Read the model definition and answer for the solid it produces. Units are mm, in the model's axes. Face numbers are marked on the shaded views. A direction names the side the tool comes from. Coordinates: 2 decimals unless noted, no trailing zeros. Write each loop counter-clockwise with the first axis right and the second up, starting at its lowest first coordinate (ties: lowest second). Pieces come first, ordered by that corner, then holes. Notation, with made-up numbers: (37, -21.5) -> (58, -21.5) arc R20 cw to (58, 6.5) -> close; hole circle Ø6 at (-30.75, 72). An arc over 180 degrees is marked (long way). One line per item, written item: value. Start each with the question number.
1. Find section C-C, the plane y = 7.5. State how many separate pieces and enclosed holes the cut face has, and give its area (3 significant figures).
2. Find section D-D, the plane x = -21.5. Write down the section's boundary in (y, z).
3. Find section B-B, the plane x = 0. Write down the section's boundary in (y, z), and give its area (3 significant figures).
4. Find section A-A, the plane z = -115. Write down the section's boundary in (x, y), and give its area (3 significant figures).
5. For a pull along Z with two mould halves and no side action, classify the marked faces 1, 2 and 3 as pulls with the +Z half, pulls with the -Z half, needs draft (parallel to the pull), parting line crosses it, or undercut.
6. Given P1, Ø1, axis at y = 7, z = -140.5, coming from the -X side; P2, Ø1, axis at x = 2.5, y = 4.5, coming from the -Z side; P3, Ø18, axis at x = 0, z = -150, coming from the -Y side; P4, Ø5, axis at y = 6.5, z = -125, coming from the +X side, each flat-ended and moving along its own axis, determine where each tip first touches the part or whether it passes through.
7. For the marked faces 4 and 5, determine the directions among +Z, -Z, +X, -X, +Y, -Y from which every point of the face is accessible in a straight line to the end or side of a thin tool.
8. Consider line 1 along X through (y, z) = (3.75, -150); line 2 along Z through (x, y) = (-12.5, 5.25); line 3 along X through (y, z) = (2, -59.5). Determine where each line is inside the solid, lowest interval first.
```python
from build123d import *

# Parameters (mm, degrees)
SKETCH_1_R               = 5
SKETCH_1_R_2             = 15
EXTRUDE_1_DEPTH          = 12
FILLET_1_R               = 3
SKETCH_2_R               = 2
CUT_EXTRUDE_1_DEPTH      = 179.881245523
PATTERN_CIRCULAR_3_COUNT = 2
PATTERN_CIRCULAR_3_ANGLE = 50
PATTERN_CIRCULAR_4_COUNT = 2
PATTERN_CIRCULAR_4_ANGLE = 50


with BuildPart() as part:
    # 草图1 → 凸台-拉伸1 (new body)
    with BuildSketch(Plane(origin=(0, 0, 0), x_dir=(1, 0, 0), z_dir=(0, 1, 0))):
        with BuildLine():
            Line((-17.971076762, -1.02), (-26.457418567, 148.498333333))
            ThreePointArc((-26.457418567, 148.498333333), (0, 176.5), (26.457418567, 148.498333333))
            Line((26.457418567, 148.498333333), (17.971076762, -1.02))
            ThreePointArc((17.971076762, -1.02), (0, -18), (-17.971076762, -1.02))
        make_face()
        with Locations(Location((0, 0, 0), (0, 0, 270))):
            Circle(SKETCH_1_R, mode=Mode.SUBTRACT)
        with Locations(Location((0, 150, 0), (0, 0, 270))):
            Circle(SKETCH_1_R_2, mode=Mode.SUBTRACT)
        Polygon((-12.740980954, 12.714849757), (-18.554385191, 115.139490738), (10.712851955, 17.329399023), align=None, mode=Mode.SUBTRACT)
        Polygon((13.283215706, 22.268322657), (18.830257334, 120), (-12, 127), align=None, mode=Mode.SUBTRACT)
    extrude(amount=EXTRUDE_1_DEPTH)

    # 圆角1
    fillet_1_edges = [part.edges().sort_by_distance(p)[0] for p in [
        (-12.740980954, 6, -12.714849757),
        (10.712851955, 6, -17.329399023),
        (-18.554385191, 6, -115.139490738),
        (18.830257334, 6, -120),
        (-12, 6, -127),
        (13.283215706, 6, -22.268322657),
    ]]
    fillet(fillet_1_edges, radius=FILLET_1_R)

    # 草图2 → 切除-拉伸1 (cut, through all)
    with BuildSketch(Plane(origin=(0, 12, 0), x_dir=(1, 0, 0), z_dir=(0, 1, 0))):
        with Locations(Location((-21.5, 150, 0), (0, 0, 270))):
            Circle(SKETCH_2_R)
        with Locations(Location((21.5, 150, 0), (0, 0, 270))):
            Circle(SKETCH_2_R)
    cut_extrude_1 = extrude(amount=-CUT_EXTRUDE_1_DEPTH, mode=Mode.SUBTRACT)

    # 阵列(圆周)3: 切除-拉伸1 ×2 about axis
    pattern_circular_3_axis = Axis((0, 0, -150), (0, 1, 0))
    for i in range(1, PATTERN_CIRCULAR_3_COUNT):
        add(cut_extrude_1.rotate(pattern_circular_3_axis, i * PATTERN_CIRCULAR_3_ANGLE / (PATTERN_CIRCULAR_3_COUNT - 1)), mode=Mode.SUBTRACT)

    # 阵列(圆周)4: 切除-拉伸1 ×2 about axis
    pattern_circular_4_axis = Axis((0, 0, -150), (0, -1, 0))
    for i in range(1, PATTERN_CIRCULAR_4_COUNT):
        add(cut_extrude_1.rotate(pattern_circular_4_axis, i * PATTERN_CIRCULAR_4_ANGLE / (PATTERN_CIRCULAR_4_COUNT - 1)), mode=Mode.SUBTRACT)


solid = part.part
```
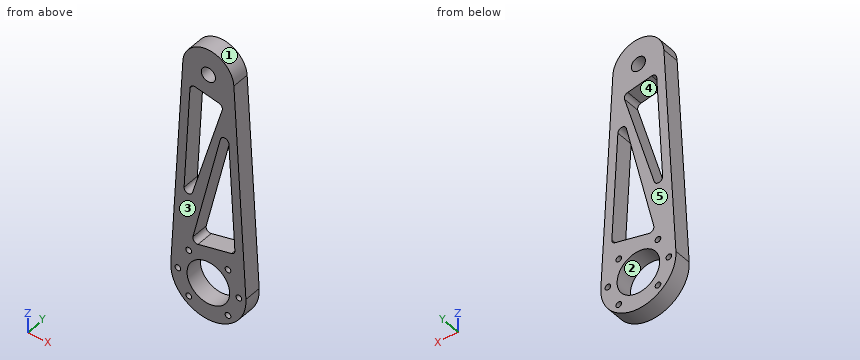
Answer block:
1. separate pieces: 1
1. enclosed holes: 10
1. area: 4,820 mm2
2. outline: (0, -165.49) -> (12, -165.49) -> (12, -152) -> (0, -152) -> close; (0, -148) -> (12, -148) -> (12, -61.16) -> (0, -61.16) -> close
3. outline: (0, -176.5) -> (12, -176.5) -> (12, -165) -> (0, -165) -> close; (0, -135) -> (12, -135) -> (12, -124.28) -> (0, -124.28) -> close; (0, -77.29) -> (12, -77.29) -> (12, -53.13) -> (0, -53.13) -> close; (0, -15.22) -> (12, -15.22) -> (12, -5) -> (0, -5) -> close; (0, 5) -> (12, 5) -> (12, 18) -> (0, 18) -> close
3. area: 835 mm2
4. outline: (-24.56, 0) -> (-9.1, 0) -> (-9.1, 12) -> (-24.56, 12) -> close; (18.55, 0) -> (24.56, 0) -> (24.56, 12) -> (18.55, 12) -> close
4. area: 258 mm2
5. face 1: pulls with the +Z half
5. face 2: undercut
5. face 3: needs draft
6. P1: stops at x = -26.03
6. P2: stops at z = -176.42
6. P3: passes through
6. P4: stops at x = 25.27
7. face 4: +Y, -Y
7. face 5: +Z, -Z, +X, -X, +Y
8. line 1: x = -26.5 to -23.5, -19.5 to -15, 15 to 19.5, 23.5 to 26.5
8. line 2: z = -173.37 to -167.97, -164.97 to -158.29, -141.71 to -135.03, -132.03 to -92.36, -14.76 to 12.95
8. line 3: x = -21.41 to -15.4, -1.91 to 4.3, 15.4 to 21.41
